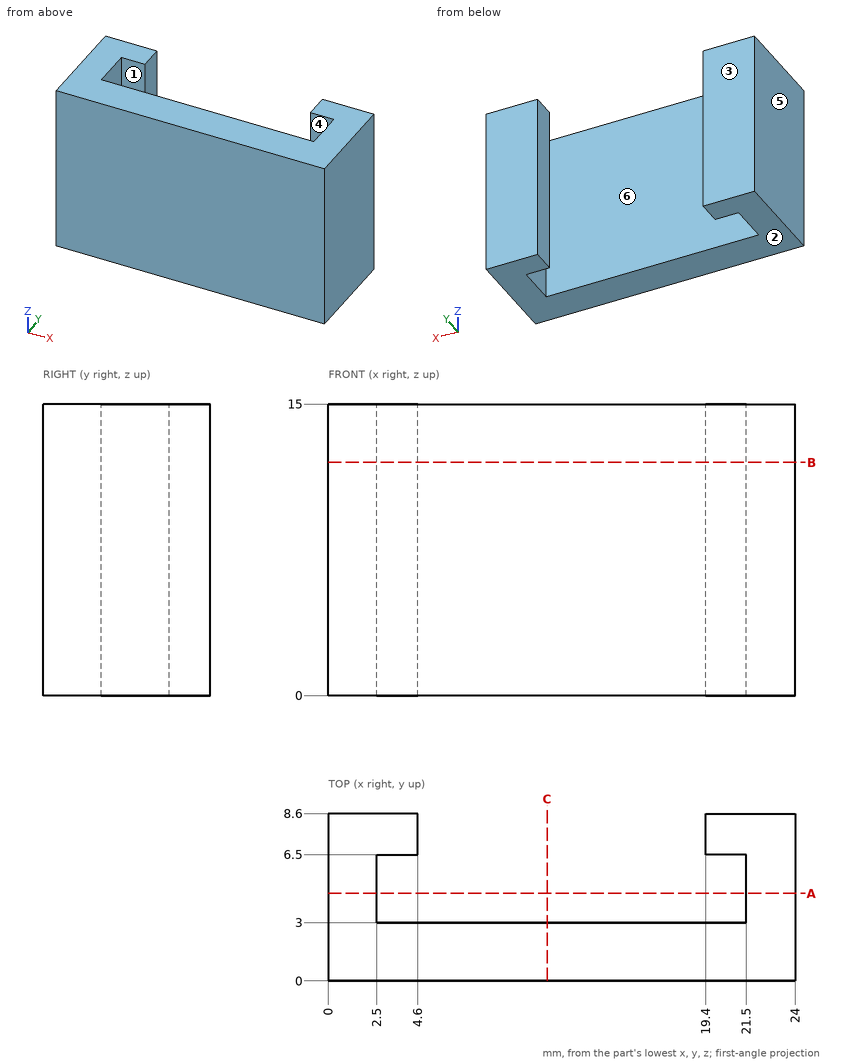
Design review of the part shown in the three views and the two pictorial views. Dimensions are in mm from the part's minimum x, y and z. A direction names the side the tool comes from. Coordinates: 2 decimals unless noted, no trailing zeros. Write each loop counter-clockwise with the first axis right and the second up, starting at its lowest first coordinate (ties: lowest second). Pieces come first, ordered by that corner, then holes. Notation, with made-up numbers: (-3.75, -16.75) -> (49.25, -16.75) arc R26 cw to (49.25, 1.25) -> close; hole circle Ø6 at (-4, 41). An arc over 180 degrees is marked (long way). Answer in a Markdown table with one row per item.
1. We need section C-C, the plane x = 11.25. State the section outline as (y, z) points, and give its area (3 significant figures).
Answers below:
| item | result |
|---|---|
| outline | (0, 0) -> (3, 0) -> (3, 15) -> (0, 15) -> close |
| area | 45.0 mm^2 |
2. Clearance check with a flat-ended pin moving along its axis: pin 1 Ø5 at (x, z) = (17, 7.5) entering from -Y. State where the tip first meets the part, or that it passes through.
Answers below:
| item | result |
|---|---|
| pin 1 | stops at y = 0 |
3. We need section A-A, the plane y = 4.5. State the section outline as (x, z) points, and give its area (3 significant figures).
Answers below:
| item | result |
|---|---|
| outline | (0, 0) -> (2.5, 0) -> (2.5, 15) -> (0, 15) -> close; (21.5, 0) -> (24, 0) -> (24, 15) -> (21.5, 15) -> close |
| area | 75.0 mm^2 |
4. For the marked faces 5 and 6, list the 3-axis set-ups (+Z, -Z, +X, -X, +Y, -Y) from which the entire face can be reached by the end or side of a thin tool; tool diameter is ignored.
Answers below:
| item | result |
|---|---|
| face 5 | +Z, -Z, -X, +Y, -Y |
| face 6 | +Z, -Z |
5. Draft analysis for pull direction Y (two halves, no side actions). For the marked faces 1, 2, 3 and 4, state which applies: +Y half, -Y half, draft (parallel to the pull), parting line (faces both ways), or undercut.
Answers below:
| item | result |
|---|---|
| face 1 | undercut |
| face 2 | draft |
| face 3 | +Y half |
| face 4 | undercut |
6. Wall thickness on probe 1 along Y at (x, z) = (20.25, 14); probe 2 along X at (y, z) = (7, 0.75); probe 3 along X at (y, z) = (4, 2): over which ranges is each line inside the solid? List them lowest first. Write a range as [from, to].
Answers below:
| item | result |
|---|---|
| probe 1 | y = [0, 3], [6.5, 8.6] |
| probe 2 | x = [0, 4.6], [19.4, 24] |
| probe 3 | x = [0, 2.5], [21.5, 24] |
7. We need section B-B, the plane z = 12. State the section outline as (x, y) points, and give its area (3 significant figures).
Answers below:
| item | result |
|---|---|
| outline | (0, 0) -> (24, 0) -> (24, 8.6) -> (19.4, 8.6) -> (19.4, 6.5) -> (21.5, 6.5) -> (21.5, 3) -> (2.5, 3) -> (2.5, 6.5) -> (4.6, 6.5) -> (4.6, 8.6) -> (0, 8.6) -> close |
| area | 109 mm^2 |
